from build123d import *

# Parameters (mm, degrees)
F1_DEPTH = 76.2


with BuildPart() as f1:
    # F0 (on Top) → F1 (new body)
    with BuildSketch(Plane.XY):
        Polygon((50.8, -50.8), (50.8, 50.8), (0, 50.8), (-50.8, 50.8), (-50.8, -50.8), align=None)
        Polygon((-44.45, 44.45), (0, 44.45), (44.45, 44.45), (44.45, 0), (44.45, -44.45), (0, -44.45), (-44.45, -44.45), (-44.45, 0), align=None, mode=Mode.SUBTRACT)
    extrude(amount=F1_DEPTH)


solid = f1.part
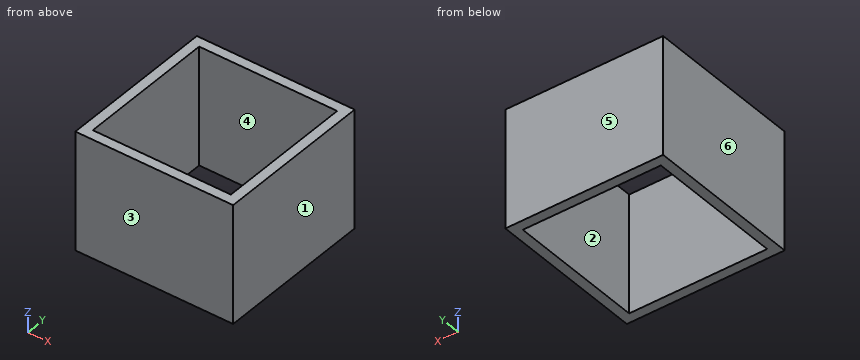
Verification items for the finished model (mm, model axes). Face numbers are marked on the shaded views. A direction names the side the tool comes from. Give positions to 0.01 mm unless a question says otherwise; leave off trailing zeros. Loops run counter-clockwise (first coordinate to the right, second up) from the corner with the lowest first, then second, coordinate; pieces in that order, holes last.
1) Thickness scan on line 1 along Y through (x, z) = (5.5, 39.5). Record the ranges inside material, lowest first.
2) Sectioned sample at A-A, the plane y = -14.5. Enter the section's corners in (x, z).
3) Draft check along Y on the marked faces 3, 4, 5 and 6. Enter one of: pulls with the +Y half, pulls with the -Y half, needs draft (parallel to the pull), parting line crosses it, or undercut.
4) Set-up check for the marked faces 1 and 2: record each of +Z, -Z, +X, -X, +Y, -Y from which the full face is reachable in a straight line by a thin tool's end or side.
5) Sectioned sample at B-B, the plane z = 28.5. Enter the section's corners in (x, y), then the cut area to 3 significant figures.
Answers:
1. line 1: y = -50.8 to -44.45, 44.45 to 50.8
2. outline: (-50.8, 0) - (-44.45, 0) - (-44.45, 76.2) - (-50.8, 76.2) - close; (44.45, 0) - (50.8, 0) - (50.8, 76.2) - (44.45, 76.2) - close
3. face 3: pulls with the -Y half
3. face 4: undercut
3. face 5: pulls with the +Y half
3. face 6: needs draft
4. face 1: +Z, -Z, +X, +Y, -Y
4. face 2: +Z, -Z
5. outline: (-50.8, -50.8) - (50.8, -50.8) - (50.8, 50.8) - (-50.8, 50.8) - close; hole (-44.45, -44.45) - (44.45, -44.45) - (44.45, 44.45) - (-44.45, 44.45) - close
5. area: 2,420 mm2
